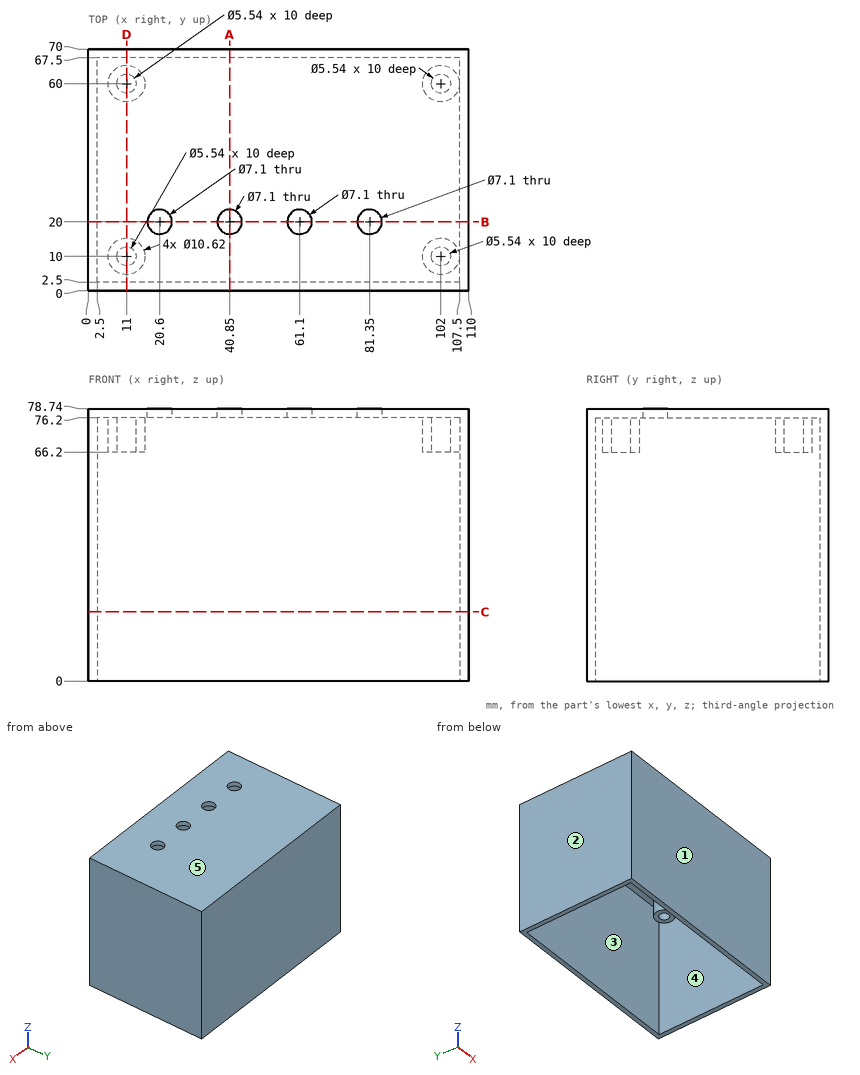
Here's the drawing with two shaded views (mm, measured from the low corner). I have some questions. A direction names the side the tool comes from. Round coordinates to 2 decimals unless told otherwise and drop trailing zeros. Loops run counter-clockwise (first coordinate to the right, second up) from the corner with the lowest first, then second, coordinate; pieces in that order, holes last. Notation, with made-up numbers: M -4.75,46 L 5.25,46 A30 ccw 5.25,77 Z; hole C 22.25,63 d11. An arc over 180 degrees is marked long. Put each result on its own line as item: value.
Q1. Thinking about a two-plate mould opening in Y: for the marked faces 1, 2 and 3, which applies, released by +Y, released by -Y, zero draft, split by the parting line, or undercut?
Check result:
face 1: released by -Y
face 2: zero draft
face 3: undercut
Q2. For pin 1 (6 mm diameter, centred on x = 41, y = 41, fed in from -Z); pin 2 (8.5 mm diameter, centred on x = 9, y = 9.5, fed in from -Z); pin 3 (6.5 mm diameter, centred on x = 61.1, y = 20, fed in from -Z), each with a flat end and sliding along its axis, tell me the tip position at first contact or that it passes through.
Check result:
pin 1: z = 76.2
pin 2: z = 66.2
pin 3: through
Q3. Imagine slicing it at A-A (x = 40.85). Write out the boundary of the cut face in (y, z), then the cut area to 3 significant figures.
Check result:
outline: M 0,0 L 2.5,0 L 2.5,76.2 L 16.45,76.2 L 16.45,78.74 L 0,78.74 Z; M 23.55,76.2 L 67.5,76.2 L 67.5,0 L 70,0 L 70,78.74 L 23.55,78.74 Z
area: 541 mm2
Q4. Imagine slicing it at B-B (y = 20). Write out the boundary of the cut face in (x, z), then the cut area to 3 significant figures.
Check result:
outline: M 0,0 L 2.5,0 L 2.5,76.2 L 17.05,76.2 L 17.05,78.74 L 0,78.74 Z; M 24.15,76.2 L 37.3,76.2 L 37.3,78.74 L 24.15,78.74 Z; M 44.4,76.2 L 57.55,76.2 L 57.55,78.74 L 44.4,78.74 Z; M 64.65,76.2 L 77.8,76.2 L 77.8,78.74 L 64.65,78.74 Z; M 84.9,76.2 L 107.5,76.2 L 107.5,0 L 110,0 L 110,78.74 L 84.9,78.74 Z
area: 588 mm2
Q5. Imagine slicing it at C-C (z = 20). Write out the boundary of the cut face in (x, y), then the cut area to 3 significant figures.
Check result:
outline: M 0,0 L 110,0 L 110,70 L 0,70 Z; hole M 2.5,2.5 L 107.5,2.5 L 107.5,67.5 L 2.5,67.5 Z
area: 875 mm2
Q6. Imagine slicing it at D-D (x = 11). Write out the boundary of the cut face in (y, z), then the cut area to 3 significant figures.
Check result:
outline: M 0,0 L 2.5,0 L 2.5,76.2 L 4.69,76.2 L 4.69,66.2 L 7.23,66.2 L 7.23,76.2 L 12.77,76.2 L 12.77,66.2 L 15.31,66.2 L 15.31,76.2 L 54.69,76.2 L 54.69,66.2 L 57.23,66.2 L 57.23,76.2 L 62.77,76.2 L 62.77,66.2 L 65.31,66.2 L 65.31,76.2 L 67.5,76.2 L 67.5,0 L 70,0 L 70,78.74 L 0,78.74 Z
area: 660 mm2
Q7. I need wall thicknesses on probe 1 along Y at (x, z) = (102, 73); probe 2 along X at (y, z) = (15.5, 75.5); probe 3 along Y at (x, z) = (40.85, 77.3). Which ranges of each line are inside material? Lowest first, please.
Check result:
probe 1: 0 to 2.5, 4.69 to 7.23, 12.77 to 15.31, 54.69 to 57.23, 62.77 to 65.31, 67.5 to 70
probe 2: 0 to 2.5, 107.5 to 110
probe 3: 0 to 16.45, 23.55 to 70
Q8. On a 3-axis mill with a long thin cutter (end or side, diameter ignored), from which of +Z, -Z, +X, -X, +Y, -Y can I reach the whole of each face in a straight line? I mean the marked faces 4 and 5. Say none if no direction works.
Check result:
face 4: -Z
face 5: +Z, +X, -X, +Y, -Y
